from build123d import *

# Parameters (mm, degrees)
PAD029_DEPTH    = 15
SKETCH081_R     = 2.25
HOLE038_DEPTH   = 26.001
POCKET053_DEPTH = 18
POCKET054_DEPTH = 6.5


with BuildPart() as part:
    # Sketch079 → Pad029 (new body)
    with BuildSketch(Plane.XY):
        with BuildLine():
            ThreePointArc((117, 103.771105), (115.5, 122.35), (114, 103.771105))
            Line((114, 103.771105), (114, 80))
            Line((106.5, 80), (114, 80))
            ThreePointArc((102.5, 84), (103.671573, 81.171573), (106.5, 80))
            Line((102.5, 113), (102.5, 84))
            ThreePointArc((128.5, 113), (115.5, 126), (102.5, 113))
            Line((128.5, 113), (128.5, 109.880832))
            ThreePointArc((124.5, 100.5), (127.458261, 104.781812), (128.5, 109.880832))
            Line((123.5, 100.5), (124.5, 100.5))
            Line((123.5, 64), (123.5, 100.5))
            Line((119, 64), (123.5, 64))
            ThreePointArc((117, 66), (117.585786, 64.585786), (119, 64))
            Line((117, 103.771105), (117, 66))
        make_face()
    extrude(amount=PAD029_DEPTH)

    # Sketch081 (on DatumPlane) → Hole038 (cut, through all)
    with BuildSketch(Plane(origin=(128.5, 0, 0), x_dir=(0, 0, 1), z_dir=(1, 0, 0))):
        with Locations((7.5, -90)):
            Circle(SKETCH081_R)
        with Locations((7.5, -74)):
            Circle(SKETCH081_R)
    extrude(amount=-HOLE038_DEPTH, mode=Mode.SUBTRACT)

    # Sketch082 (on DatumPlane) → Pocket053 (cut)
    with BuildSketch(Plane(origin=(102.5, 0, 0), x_dir=(0, -1, 0), z_dir=(-1, 0, 0))):
        Polygon((-69.785343, 7.5), (-71.892672, 11.15), (-76.107328, 11.15), (-78.214657, 7.5), (-76.107328, 3.85), (-71.892672, 3.85), align=None)
    extrude(amount=-POCKET053_DEPTH, mode=Mode.SUBTRACT)

    # Sketch083 (on DatumPlane) → Pocket054 (cut)
    with BuildSketch(Plane(origin=(102.5, 0, 0), x_dir=(0, -1, 0), z_dir=(-1, 0, 0))):
        Polygon((-85.785343, 7.5), (-87.892672, 11.15), (-92.107328, 11.15), (-94.214657, 7.5), (-92.107328, 3.85), (-87.892672, 3.85), align=None)
    extrude(amount=-POCKET054_DEPTH, mode=Mode.SUBTRACT)


with BuildPart() as part_1:
    # Body022006 placement: moved
    add(part.part.moved(Location((-2.5, 0, 770))))


solid = part_1.part
Input: part model. Units: mm. Frame: model coordinates. A direction names the side the tool comes from. Give positions to 0.01 mm unless a question says otherwise; leave off trailing zeros. Order: outer loops, then holes, each group sorted by start corner. A loop starts at its lowest first (then second) coordinate and runs counter-clockwise, first axis right, second up.
Q1. Draft query along Y for faces 1 (the cylindrical face through (117.796, 89.324, 779.646)), 2 (the flat face through (110, 95, 770)), 3 (the flat face through (103.204, 86.854, 775.649)), 4 (the flat face through (108, 80, 777)). Return one class per face: +Y half, -Y half, draft (parallel to the pull), parting line (faces both ways), or undercut.
Checked values:
face 1: undercut
face 2: draft
face 3: undercut
face 4: -Y half
Q2. Set-up query: faces 5 (the flat face through (116, 74, 773.85)), 6 (the flat face through (111.5, 92, 776)), 7 (the flat face through (121, 82, 777)). Return all of +Z, -Z, +X, -X, +Y, -Y with unobstructed straight access to the full face (end or side cutting, diameter ignored); none if empty.
Checked values:
face 5: -X
face 6: +Z, -Z, -Y
face 7: +Z, -Z, +X, -Y
Q3. Section D-D on z = 771.25. Output: boundary loops of the cut face in (x, y).
Checked values:
outline: (100, 84) arc R4 ccw to (104, 80) - (111.5, 80) - (111.5, 103.77) arc R9.35 cw (long way) to (114.5, 103.77) - (114.5, 66) arc R2 ccw to (116.5, 64) - (121, 64) - (121, 100.5) - (122, 100.5) arc R13 ccw to (126, 109.88) - (126, 113) arc R13 ccw to (100, 113) - close
Q4. Section C-C on x = 118.75. Output: boundary loops of the cut face in (y, z).
Checked values:
outline: (64, 770) - (105.63, 770) - (105.63, 785) - (64, 785) - close; (120.37, 770) - (124.66, 770) - (124.66, 785) - (120.37, 785) - close; hole circle Ø4.5 at (74, 777.5); hole circle Ø4.5 at (90, 777.5)
Q5. Section B-B on x = 109. Output: boundary loops of the cut face in (y, z).
Checked values:
outline: (80, 770) - (104.55, 770) - (104.55, 785) - (80, 785) - close; (121.45, 770) - (125.37, 770) - (125.37, 785) - (121.45, 785) - close; hole circle Ø4.5 at (90, 777.5)
Q6. Section A-A on y = 98.5. Output: boundary loops of the cut face in (x, z).
Checked values:
outline: (100, 770) - (111.5, 770) - (111.5, 785) - (100, 785) - close; (114.5, 770) - (121, 770) - (121, 785) - (114.5, 785) - close
Q7. Contact query for flat-ended pins moving along their axis: pin 1 Ø7.5 at (y, z) = (89.5, 775) entering from +X; pin 2 Ø2 at (x, z) = (111.5, 778.5) entering from +Y; pin 3 Ø6 at (y, z) = (74, 777.5) entering from -X. Output: stop coordinate, or through.
Checked values:
pin 1: stops at x = 121
pin 2: stops at y = 125.99
pin 3: stops at x = 118
Q8. Ray query, probe 1 along X at (y, z) = (99.5, 773.75); probe 2 along Y at (x, z) = (120.15, 777.5); probe 3 along Z at (x, y) = (118.75, 90). Return the intervals inside material, ascending.
Checked values:
probe 1: x = 100 to 111.5, 114.5 to 121
probe 2: y = 64 to 71.75, 76.25 to 87.75, 92.25 to 106.98, 119.02 to 123.86
probe 3: z = 770 to 775.25, 779.75 to 785
